Input: part model. Units: mm. Frame: model coordinates. A direction names the side the tool comes from. Give positions to 0.01 mm unless a question says otherwise; leave off trailing zeros. Loops run counter-clockwise (first coordinate to the right, second up) from the corner with the lowest first, then second, coordinate; pieces in that order, holes last. Notation, with made-up numbers: (-23.5, -22) -> (16.5, -22) arc R13 ccw to (16.5, 0) -> close; hole circle Ø8 at (60.25, -2.75). An arc over 180 degrees is marked (long way). One line per question, with ' | ' between items.
from build123d import *

# Parameters (mm, degrees)
SKETCH15_W         = 290
SKETCH15_H         = 240
BASE_FLANGE1_DEPTH = 3
EDGE_FLANGE1_DEPTH = 240
EDGE_FLANGE2_DEPTH = 290
EDGE_FLANGE3_DEPTH = 240
EDGE_FLANGE4_DEPTH = 290
SKETCH32_R         = 3.15
CUT_EXTRUDE3_DEPTH = 386.680145843
SKETCH33_R         = 6
CUT_EXTRUDE4_DEPTH = 10


# Sheet-metal steps are written as plain solids
with BuildPart() as part:
    # Sketch15 → Base-Flange1 (new body)
    with BuildSketch(Plane(origin=(0, 0, 0), x_dir=(1, 0, 0), z_dir=(0, 1, 0))):
        with Locations((145, 120)):
            Rectangle(SKETCH15_W, SKETCH15_H)
    extrude(amount=-BASE_FLANGE1_DEPTH)

    # Edge-Flange1 section (across the edge) → Edge-Flange1 (add)
    with BuildSketch(Plane(origin=(-0.7366, 0, -240), x_dir=(1, 0, 0), z_dir=(0, 0, 1))):
        with BuildLine():
            Line((-3, 0.7366), (-3, 35))
            Line((-3, 35), (0, 35))
            Line((0, 35), (0, 0.7366))
            ThreePointArc((0, 0.7366), (0.215745145, 0.215745145), (0.7366, 0))
            Line((0.7366, 0), (0.7366, -3))
            ThreePointArc((0.7366, -3), (-1.905575199, -1.905575199), (-3, 0.7366))
        make_face()
    extrude(amount=EDGE_FLANGE1_DEPTH)

    # Edge-Flange2 section (across the edge) → Edge-Flange2 (add)
    with BuildSketch(Plane(origin=(0, 0, 0.7366), x_dir=(0, 0, -1), z_dir=(1, 0, 0))):
        with BuildLine():
            Line((-3, 0.7366), (-3, 35))
            Line((-3, 35), (0, 35))
            Line((0, 35), (0, 0.7366))
            ThreePointArc((0, 0.7366), (0.215745145, 0.215745145), (0.7366, 0))
            Line((0.7366, 0), (0.7366, -3))
            ThreePointArc((0.7366, -3), (-1.905575199, -1.905575199), (-3, 0.7366))
        make_face()
    extrude(amount=EDGE_FLANGE2_DEPTH)

    # Edge-Flange3 section (across the edge) → Edge-Flange3 (add)
    with BuildSketch(Plane(origin=(290.7366, 0, 0), x_dir=(-1, 0, 0), z_dir=(0, 0, -1))):
        with BuildLine():
            Line((-3, 0.7366), (-3, 35))
            Line((-3, 35), (0, 35))
            Line((0, 35), (0, 0.7366))
            ThreePointArc((0, 0.7366), (0.215745145, 0.215745145), (0.7366, 0))
            Line((0.7366, 0), (0.7366, -3))
            ThreePointArc((0.7366, -3), (-1.905575199, -1.905575199), (-3, 0.7366))
        make_face()
    extrude(amount=EDGE_FLANGE3_DEPTH)

    # Edge-Flange4 section (across the edge) → Edge-Flange4 (add)
    with BuildSketch(Plane(origin=(290, 0, -240.7366), x_dir=(0, 0, 1), z_dir=(-1, 0, 0))):
        with BuildLine():
            Line((-3, 0.7366), (-3, 35))
            Line((-3, 35), (0, 35))
            Line((0, 35), (0, 0.7366))
            ThreePointArc((0, 0.7366), (0.215745145, 0.215745145), (0.7366, 0))
            Line((0.7366, 0), (0.7366, -3))
            ThreePointArc((0.7366, -3), (-1.905575199, -1.905575199), (-3, 0.7366))
        make_face()
    extrude(amount=EDGE_FLANGE4_DEPTH)

    # Sketch32 → Cut-Extrude3 (cut, through all)
    with BuildSketch(Plane.XY.offset(3.7366)):
        with Locations((16.2634, 17)):
            Circle(SKETCH32_R)
        with Locations((28.2634, 17)):
            Circle(SKETCH32_R)
        with Locations((40.2634, 17)):
            Circle(SKETCH32_R)
        with Locations((52.2634, 17)):
            Circle(SKETCH32_R)
        with Locations((64.2634, 17)):
            Circle(SKETCH32_R)
        with Locations((76.2634, 17)):
            Circle(SKETCH32_R)
        with Locations((88.2634, 17)):
            Circle(SKETCH32_R)
        with Locations((100.2634, 17)):
            Circle(SKETCH32_R)
        with Locations((112.2634, 17)):
            Circle(SKETCH32_R)
        with Locations((124.2634, 17)):
            Circle(SKETCH32_R)
    extrude(amount=-CUT_EXTRUDE3_DEPTH, mode=Mode.SUBTRACT)

    # Sketch33 → Cut-Extrude4 (cut)
    with BuildSketch(Plane.XY.offset(3.7366)):
        with Locations((169.2634, 17)):
            Circle(SKETCH33_R)
        with Locations((209.2634, 17)):
            Circle(SKETCH33_R)
    extrude(amount=-CUT_EXTRUDE4_DEPTH, mode=Mode.SUBTRACT)


solid = part.part
1. Pin query (flat end, axial travel): P1, Ø2, axis at x = 255.5, z = -162.5, coming from the +Y side; P2, Ø1.9, axis at x = 292, y = 18.5, coming from the -Z side; P3, Ø1.1, axis at y = 14.5, z = 2, coming from the -X side. Return the tip coordinate at first contact, or that it passes through.
Determined:
P1: stops at y = 0 | P2: stops at z = -240 | P3: stops at x = 0
2. Ray query, line 1 along Z through (x, y) = (11, 0.5); line 2 along X through (y, z) = (5, -210); line 3 along Y through (x, z) = (148.5, -200). Return the intervals inside material, ascending. Write a range as from..to.
Determined:
line 1: z = -243.73..-240.7, 0.7..3.73 | line 2: x = -3.74..-0.74, 290.74..293.74 | line 3: y = -3..0
3. Section query A-A (y = 7.5). Output: boundary loops of the cut face in (x, z).
Determined:
outline: (-3.74, -240) -> (-0.74, -240) -> (-0.74, 0) -> (-3.74, 0) -> close; (0, -243.74) -> (290, -243.74) -> (290, -240.74) -> (0, -240.74) -> close; (0, 0.74) -> (290, 0.74) -> (290, 3.74) -> (0, 3.74) -> close; (290.74, -240) -> (293.74, -240) -> (293.74, 0) -> (290.74, 0) -> close
4. Section query B-B (z = -188). Output: boundary loops of the cut face in (x, y).
Determined:
outline: (-3.74, 0.74) arc R3.74 ccw to (0, -3) -> (290, -3) arc R3.74 ccw to (293.74, 0.74) -> (293.74, 35) -> (290.74, 35) -> (290.74, 0.74) arc R0.74 cw to (290, 0) -> (0, 0) arc R0.74 cw to (-0.74, 0.74) -> (-0.74, 35) -> (-3.74, 35) -> close
5. Section query C-C (x = 248.5). Output: boundary loops of the cut face in (y, z).
Determined:
outline: (-3, -240) arc R3.74 ccw to (0.74, -243.74) -> (35, -243.74) -> (35, -240.74) -> (0.74, -240.74) arc R0.74 cw to (0, -240) -> (0, 0) arc R0.74 cw to (0.74, 0.74) -> (35, 0.74) -> (35, 3.74) -> (0.74, 3.74) arc R3.74 ccw to (-3, 0) -> close
6. Pull-direction query (Y, two-part tool) for faces 6 (the cylindrical face through (73.116, 17.138, -242.216)), 7 (the flat face through (143, 0, -122)), 8 (the flat face through (143, 18, 0.737)); classes: pulls with the +Y half, pulls with the -Y half, needs draft (parallel to the pull), parting line crosses it, or undercut.
Determined:
face 6: undercut | face 7: pulls with the +Y half | face 8: needs draft
7. Reachability of faces 1 (the cylindrical face through (163.27, 17.26, 2.26)), 2 (the flat face through (143, 18, 3.737)), 3 (the cylindrical face through (61.764, 15.083, -242.216)), 4 (the flat face through (290.737, 18, -118)), 5 (the flat face through (147, 18, -240.737)) from +Z, -Z, +X, -X, +Y, -Y: full face, straight path, thin tool, end or side. Return the list, or none.
Determined:
face 1: +Z | face 2: +Z, +X, -X, +Y, -Y | face 3: +Z, -Z | face 4: +Z, -Z, +Y | face 5: +X, -X, +Y
